Autodesk Inventor part; units mm, degrees
ref_plane "YZ Plane" through (0, 0, 0) normal (1, 0, 0) x (0, 1, 0)
ref_plane "XZ Plane" through (0, 0, 0) normal (0, 1, 0) x (-1, 0, 0)
ref_plane "XY Plane" through (0, 0, 0) normal (0, 0, 1) x (1, 0, 0)
sketch "Sketch2" plane through (0, 0, 0) normal (0, 0, 1) x (1, 0, 0)
  line L0 (0, 0) -> (0, 5.2095) construction
  circle A0 centre (0, 29.7999) radius 10.2397 construction
  arc A1 (-8.9837, 19.5602) -> (-10.7158, 16.5602) centre (-8.9837, 17.5602) ccw
  line L1 (-8.9837, 19.5602) -> (8.9837, 19.5602)
  arc A2 (10.7158, 16.5602) -> (8.9837, 19.5602) centre (8.9837, 17.5602) ccw
  line L2 (-10.7158, 16.5602) -> (-1.7321, 1)
  line L3 (10.7158, 16.5602) -> (1.7321, 1)
  arc A3 (-1.7321, 1) -> (1.7321, 1) centre (0, 2) ccw
  line L4 (-25, -4.5) -> (25, -4.5) construction
  line L5 (-23.95, -3) -> (-23.95, -6) construction
  line L6 (-25, -3) -> (-25, -6)
  line L7 (-22.9, -6) -> (-22.9, -3) construction
  arc A4 (-22.9, -3) -> (-25, -3) centre (-23.95, -3) ccw
  arc A5 (-25, -6) -> (-22.9, -6) centre (-23.95, -6) ccw
  arc A6 (25, -3) -> (22.9, -3) centre (23.95, -3) ccw
  line L8 (25, -3) -> (25, -6)
  arc A7 (22.9, -6) -> (25, -6) centre (23.95, -6) ccw
  line L9 (16.3793, 15.3817) -> (28.6251, 3.4314)
  arc A8 (27.2282, 0) -> (28.6251, 3.4314) centre (27.2282, 2) ccw
  line L10 (27.2282, 0) -> (8.0829, 0)
  line L11 (-25, -3) -> (-23.95, -3) construction
  line L12 (-22.9, -3) -> (22.9, -3)
  line L13 (-25, -6) -> (-23.95, -6) construction
  line L14 (-22.9, -6) -> (22.9, -6)
  line L15 (-26.5636, -1.95) -> (-22.5758, -1.95) construction
  line L16 (14.2621, -9) -> (0, -9)
  line L17 (-16.3793, 15.3817) -> (-28.6251, 3.4314)
  line L18 (-27.2282, 0) -> (-8.0829, 0)
  arc A9 (-28.6251, 3.4314) -> (-27.2282, 0) centre (-27.2282, 2) ccw
  line L19 (-14.2621, -9) -> (0, -9)
  arc A10 (16.3793, 15.3817) -> (13.2504, 14.9503) centre (14.9824, 13.9503) ccw
  line L20 (13.2504, 14.9503) -> (6.3509, 3)
  arc A11 (6.3509, 3) -> (8.0829, 0) centre (8.0829, 2) ccw
  arc A12 (-13.2504, 14.9503) -> (-16.3793, 15.3817) centre (-14.9824, 13.9503) ccw
  line L21 (-13.2504, 14.9503) -> (-6.3509, 3)
  arc A13 (-8.0829, 0) -> (-6.3509, 3) centre (-8.0829, 2) ccw
  circle A14 centre (16.5506, 23.3453) radius 7.525
  circle A15 centre (15.5646, 38.363) radius 7.525
  line L22 (34.0353, 7.514) -> (38.0125, 5.2178)
  circle A16 centre (41.3199, -13) radius 7.525
  line L23 (15.5646, 45.888) -> (7.3682, 45.888)
  line L24 (-15.5646, 45.888) -> (7.3682, 45.888)
  line L25 (-14.2621, -9) -> (0, -9)
  circle A17 centre (35, 0) radius 1.5
  circle A18 centre (35, 0) radius 3.025
  circle A19 centre (35, 0) radius 6.025
  circle A20 centre (-35, 0) radius 6.025
  circle A21 centre (-35, 0) radius 3.025
  circle A22 centre (-35, 0) radius 1.5
  circle A23 centre (16.5506, 23.3453) radius 3.025
  circle A24 centre (41.3199, -13) radius 3.025
  line L26 (47.7096, -9.0254) -> (40.116, 3.1823)
  line L27 (-20.812, -60) -> (26.178, -60)
  circle A25 centre (-6, 80) radius 5.025
  circle A26 centre (-6, 80) radius 8.025
  arc A27 (35.8939, -18.2139) -> (14.2621, -9) centre (14.2621, -39) ccw
  circle A28 centre (0, 29.7999) radius 8.2397
  arc A29 (26.1288, 47.4363) -> (20.0049, 23.2712) centre (35.6549, 32.1637) ccw construction
  line L28 (22.3769, 18.583) -> (19.6218, 23.982) construction
  arc A30 (61.1577, -34.4951) -> (56.1103, -14.552) centre (52.6424, -26.04) ccw construction
  arc A31 (61.1577, -34.4951) -> (60.8311, -36.8802) centre (62.5769, -35.9043) ccw construction
  arc A32 (60.8311, -36.8802) -> (78.0598, -53.6221) centre (97.4928, -16.3882) ccw construction
  arc A33 (53.2941, -13.5379) -> (56.1103, -14.552) centre (64.3583, 12.7718) ccw construction
  arc A34 (26.0209, 0.9091) -> (22.8953, 17.5672) centre (-3.8265, 3.9311) ccw construction
  arc A35 (53.2941, -13.5379) -> (34.3508, -9.0016) centre (30.0348, -68.8462) ccw construction
  circle A36 centre (15.5646, 38.363) radius 1.5
  circle A37 centre (15.5646, 38.363) radius 3.025
  line L29 (23.0735, 38.856) -> (24.0594, 23.8383)
  circle A38 centre (16.5506, 23.3453) radius 1.5
  circle A39 centre (41.3199, -13) radius 1.5
  circle A40 centre (-41.3199, -13) radius 7.525
  circle A41 centre (-41.3199, -13) radius 3.025
  circle A42 centre (-41.3199, -13) radius 1.5
  circle A43 centre (-35, 0) radius 6.025
  circle A44 centre (-35, 0) radius 3.025
  circle A45 centre (-35, 0) radius 1.5
  circle A46 centre (-16.5506, 23.3453) radius 7.525
  circle A47 centre (-16.5506, 23.3453) radius 1.5
  circle A48 centre (-16.5506, 23.3453) radius 3.025
  circle A49 centre (-15.5646, 38.363) radius 7.525
  circle A50 centre (-15.5646, 38.363) radius 3.025
  circle A51 centre (-15.5646, 38.363) radius 1.5
  arc A52 (-14.2621, -9) -> (-35.8939, -18.2139) centre (-14.2621, -39) ccw
  line L30 (-47.7096, -9.0254) -> (-40.116, 3.1823)
  line L31 (-34.0353, 7.514) -> (-38.0125, 5.2178)
  line L32 (-23.0735, 38.856) -> (-24.0594, 23.8383)
  arc A53 (24.0646, 23.7525) -> (34.0353, 7.514) centre (44.0353, 24.8346) ccw
  arc A54 (-34.0353, 7.514) -> (-24.0646, 23.7525) centre (-44.0353, 24.8346) ccw
  circle A55 centre (35.0898, 32.1644) radius 1.25
  circle A56 centre (35.0898, 32.1644) radius 4.25
  line L33 (35.0898, 32.1644) -> (22.0882, 32.1644) construction
  line L34 (29.4054, 33.6644) -> (26.2238, 33.6644)
  arc A57 (29.4054, 33.6644) -> (31.7576, 34.8023) centre (29.4054, 36.6644) ccw
  arc A58 (23.2303, 36.4678) -> (26.2238, 33.6644) centre (26.2238, 36.6644) ccw
  line L35 (26.9132, 29.1644) -> (31.4681, 29.1644)
  line L36 (35.0898, 32.1644) -> (35.0898, 8.7801) construction
  arc A59 (33.0898, 27.5427) -> (31.4681, 29.1644) centre (31.4681, 27.5427) ccw
  line L37 (33.0898, 27.5427) -> (33.0898, 15.1122)
  arc A60 (26.9132, 29.1644) -> (23.9196, 25.9678) centre (26.9132, 26.1644) ccw
  arc A61 (27.6288, 13.3965) -> (33.0898, 15.1122) centre (30.0898, 15.1122) ccw
  line L38 (37.0898, 26.9144) -> (37.0898, 8.4431)
  arc A62 (37.0898, 8.4431) -> (38.8745, 4.614) centre (42.0898, 8.4431) ccw
  arc A63 (38.0208, 29.0868) -> (37.0898, 26.9144) centre (40.0898, 26.9144) ccw
  arc A64 (-38.8745, 4.614) -> (-37.0898, 8.4431) centre (-42.0898, 8.4431) ccw
  line L39 (-37.0898, 26.9144) -> (-37.0898, 8.4431)
  arc A65 (-33.0898, 15.1122) -> (-27.6288, 13.3965) centre (-30.0898, 15.1122) ccw
  line L40 (-33.0898, 27.5427) -> (-33.0898, 15.1122)
  circle A66 centre (-35.0898, 32.1644) radius 4.25
  arc A67 (-37.0898, 26.9144) -> (-38.0208, 29.0868) centre (-40.0898, 26.9144) ccw
  arc A68 (-31.4681, 29.1644) -> (-33.0898, 27.5427) centre (-31.4681, 27.5427) ccw
  line L41 (-26.9132, 29.1644) -> (-31.4681, 29.1644)
  arc A69 (-23.9196, 25.9678) -> (-26.9132, 29.1644) centre (-26.9132, 26.1644) ccw
  arc A70 (-26.2238, 33.6644) -> (-23.2303, 36.4678) centre (-26.2238, 36.6644) ccw
  line L42 (-29.4054, 33.6644) -> (-26.2238, 33.6644)
  arc A71 (-31.7576, 34.8023) -> (-29.4054, 33.6644) centre (-29.4054, 36.6644) ccw
  circle A72 centre (-35.0898, 32.1644) radius 1.25
  line L43 (-13.8418, 81.705) -> (-22.9178, 39.9618)
  line L44 (1.1649, 83.6145) -> (22.2831, 41.7523)
  point P0 (-23.95, -4.5)
  point P1 (0, 0)
  point P2 (-38.8745, 4.614)
  point P3 (-40.116, 3.1823)
  point P4 (-35.8939, -18.2139)
  point P5 (-27.6288, 13.3965)
  dimension "d361" = 2
  dimension "d362" = 2
  dimension "d363" = 30
  dimension "d364" = 2
  dimension "d365" = 50
  dimension "d366" = 3
  dimension "d367" = 2.1
  dimension "d368" = 25
  dimension "d369" = 2
  dimension "d370" = 60
  dimension "d371" = 3
  dimension "d372" = 2
  dimension "d373" = 2
  dimension "d374" = 3
  dimension "d375" = 3
  dimension "d376" = 6.05
  dimension "d377" = 3
  dimension "d378" = 30
  dimension "d379" = 6.05
  dimension "d380" = 6.05
  dimension "d381" = 60
  dimension "d382" = 10.05
  dimension "d383" = 3
  dimension "d384" = 4.5
  dimension "d385" = 30
  dimension "d386" = 2
  dimension "d387" = 3
  dimension "d388" = 6.05
  dimension "d389" = 4.5
  dimension "d390" = 4.5
  dimension "d391" = 4.5
  dimension "d392" = 13
  dimension "d393" = 3
  dimension "d394" = 3
  dimension "d395" = 20
  dimension "d396" = 6
  dimension "d397" = 80
  dimension "d398" = 2.5
  dimension "d399" = 3
  dimension "d400" = 1.5
  dimension "d401" = 3
  dimension "d402" = 3
  dimension "d403" = 2
  dimension "d404" = 3
  dimension "d405" = 3
  dimension "d406" = 3
  dimension "d407" = 5
  dimension "d408" = 2
  dimension "d409" = 3
extrude "Extrusion7" add sketch "Sketch2" against normal blind 3 contours A1 A46 A49 L24 L23 A15 A14 A2 L1 | A1 L2 A3 L3 A2 A14 A10 L20 A11 L10 A8 A19 L26 A16 A27 L16 L19 A52 A40 L30 A20 A9 L18 A13 L21 A12 A46 | A46 | A12 L17 A9 A20 L31 A54 A46 | A14 | A46 L32 A49 | A49 | A15 L29 A14 | A15 | A14 A53 L22 A19 A8 L9 A10 | A54 L31 A20 A64 L39 A67 A66 A68 L40 A65 | L23 L24 A49 L43 A26 L44 A15 | A20 | A69 L41 A68 A66 A71 L42 A70 L32 | L29 A58 L34 A57 A56 A59 L35 A60 | A26 | A61 L37 A59 A56 A63 L38 A62 A19 L22 A53 | A19 | A66 | A40 | A56 | A16
extrude "Extrusion8" add sketch "Sketch2" against normal blind 2 contours A18 | A21 | A23 | A24 | A37 | A41 | A48 | A50
properties part number "中間ユニット内" material "Aluminum 2014-T6"
The listing builds one solid part. Answer for the finished solid, in the listing's coordinates (mm). A direction names the side the tool comes from. Coordinates: 2 decimals unless noted, no trailing zeros. Write each loop counter-clockwise with the first axis right and the second up, starting at its lowest first coordinate (ties: lowest second). Pieces come first, ordered by that corner, then holes. Notation, with made-up numbers: M 54.25,48 L 60.25,48 A24 cw 60.25,82 Z; hole C 81,27.25 d2. An arc over 180 degrees is marked long. Use one line per item in the form item = value.
Item 1: Given P1, Ø1.5, axis at y = 48.5, z = -1.5, coming from the -X side; P2, Ø1.8, axis at x = -40.5, y = -13.5, coming from the -Z side; P3, Ø1, axis at y = 7, z = -1.5, coming from the +X side, each flat-ended and moving along its own axis, determine where each tip first touches the part or whether it passes through.
Model answer:
P1 = -21.22
P2 = -2
P3 = 37.48
Item 2: Find section A-A, the plane y = -13. Give the vertices of the cut face in (x, z).
Model answer:
outline = M -48.84,-3 L -44.34,-3 L -44.34,-2 L -42.82,-2 L -42.82,0 L -48.84,0 Z; M -39.82,-2 L -38.29,-2 L -38.29,-3 L -29.23,-3 L -29.23,0 L -39.82,0 Z; M 29.23,-3 L 38.29,-3 L 38.29,-2 L 39.82,-2 L 39.82,0 L 29.23,0 Z; M 42.82,-2 L 44.34,-2 L 44.34,-3 L 48.84,-3 L 48.84,0 L 42.82,0 Z
Item 3: Find section B-B, the plane z = -1.5. Give the number of separate pieces and of enclosed holes in the cut face, plus the area to 3 significant figures.
Model answer:
separate_pieces = 1
enclosed_holes = 18
area = 3,950 mm2
Item 4: For faces 4 (the face through (0, -6, -1)), 5 (the face through (36.3, -1.3, -2)), 6 (the face through (-23.15, 37.68, -1.48)), determine the directions among +Z, -Z, +X, -X, +Y, -Y from which every point of the face is accessible in a straight line to the end or side of a thin tool.
Model answer:
face_4 = +Z, -Z
face_5 = -Z
face_6 = +Z, -Z, -X, +Y
Item 5: The mould has two halves that part along Y. Classify faces 1 (the face through (43.97, -3.01, -1.48)), 2 (the face through (31.978, 0.133, -2.493)), 3 (the face through (10, 22, -3)): released by +Y, released by -Y, zero draft, split by the parting line, or undercut.
Model answer:
face_1 = released by +Y
face_2 = undercut
face_3 = zero draft
Item 6: Find the intervals of material crossed by probe 1 along Y at (x, z) = (6.5, -0.3); probe 2 along Y at (x, z) = (7.5, -0.4); probe 3 along Y at (x, z) = (-13, -2.2), in increasing order.
Model answer:
probe_1 = -9 to -6, -3 to 0.78, 3.26 to 9.26, 19.56 to 24.74, 34.86 to 73.04
probe_2 = -9 to -6, -3 to 0.09, 4.99 to 10.99, 19.56 to 26.39, 33.21 to 71.06
probe_3 = -9 to -6, -3 to 0, 14.52 to 36.76, 39.97 to 83.92
